The drawing under review shows one solid part. Ordinate dimensions are in mm from its lowest x, y, z. A direction names the side the tool comes from. Round coordinates to 2 decimals unless told otherwise and drop trailing zeros. Loops run counter-clockwise (first coordinate to the right, second up) from the corner with the lowest first, then second, coordinate; pieces in that order, holes last. Notation, with made-up numbers: (53.5, -24.75) -> (67.5, -24.75) arc R6 cw to (67.5, -15.75) -> close; hole circle Ø7 at (73, -13.75). An arc over 180 degrees is marked (long way). Use a Markdown table: item, result. Add a question column.
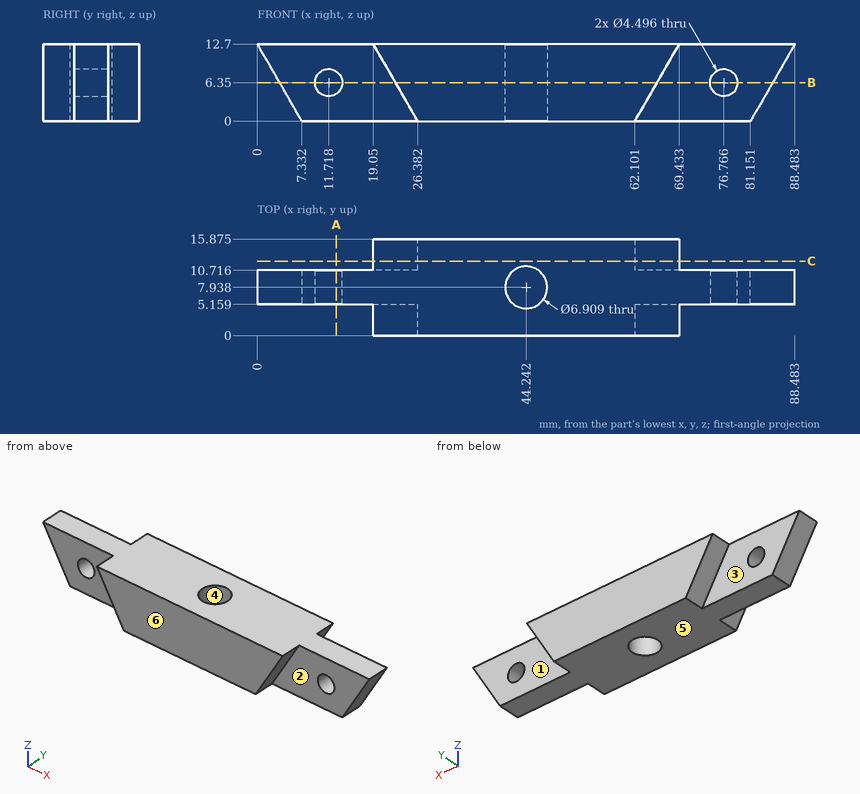
1. Insertion check: P1, Ø2, axis at x = 16, z = 7, coming from the +Y side; P2, Ø1, axis at y = 2.5, z = 10, coming from the +X side; P3, Ø1, axis at y = 7, z = 4, coming from the -X side (1 decimal). Each pin has a flat end and moves straight along its axis. Give the tip position at first contact, or say it passes through.
2. Consider section C-C on y = 12.25. State the section outline as (x, z) points, plus the area to 3 significant figures.
3. Consider section B-B on z = 6.35. State the section outline as (x, y) points (1 decimal).
4. To check wall thickness, follow probe 1 along X at (y, z) = (10, 6) (1 decimal); probe 2 along Y at (x, z) = (82, 3.75) (1 decimal); probe 3 along X at (y, z) = (9.5, 10) (1 decimal). State the ranges of each line that lie inside material, in increasing order. Write a range as from..to.
5. Consider section A-A on x = 13. State the section outline as (y, z) points (1 decimal).
6. Mouldability with a two-part tool opening along Y and no side actions: class the marked faces 4, 5 and 6 as +Y half, -Y half, draft (parallel to the pull), parting line (faces both ways), or undercut.
7. For the marked faces 1, 2 and 3, list the 3-axis set-ups (+Z, -Z, +X, -X, +Y, -Y) from which the entire face can be reached by the end or side of a thin tool; tool diameter is ignored.
Verdict:
| question | item | result |
|---|---|---|
| 1 | P1 | stops at y = 10.72 |
| 1 | P2 | stops at x = 68.16 |
| 1 | P3 | stops at x = 4.7 |
| 2 | outline | (19.05, 12.7) -> (26.38, 0) -> (62.1, 0) -> (69.43, 12.7) -> close |
| 2 | area | 547 mm² |
| 3 | outline | (3.7, 5.2) -> (9.5, 5.2) -> (9.5, 10.7) -> (3.7, 10.7) -> close; (14, 5.2) -> (22.7, 5.2) -> (22.7, 0) -> (65.8, 0) -> (65.8, 5.2) -> (74.5, 5.2) -> (74.5, 10.7) -> (65.8, 10.7) -> (65.8, 15.9) -> (22.7, 15.9) -> (22.7, 10.7) -> (14, 10.7) -> close; (79, 5.2) -> (84.8, 5.2) -> (84.8, 10.7) -> (79, 10.7) -> close; hole circle Ø6.9 at (44.2, 7.9) |
| 4 | probe 1 | x = 3.9..9.5, 13.9..41.5, 47..74.5, 79..84.6 |
| 4 | probe 2 | y = 5.2..10.7 |
| 4 | probe 3 | x = 1.6..41.2, 47.3..86.9 |
| 5 | outline | (5.2, 0) -> (10.7, 0) -> (10.7, 4.5) -> (5.2, 4.5) -> close; (5.2, 8.2) -> (10.7, 8.2) -> (10.7, 12.7) -> (5.2, 12.7) -> close |
| 6 | face 4 | undercut |
| 6 | face 5 | draft |
| 6 | face 6 | -Y half |
| 7 | face 1 | -Z, +X, +Y |
| 7 | face 2 | -Z, +X, -Y |
| 7 | face 3 | -Z, -X, +Y |
